Source: CAD feature listing. Evaluate the final solid. Frame: model axes, mm. Face numbers are marked on the shaded views. A direction names the side the tool comes from. Coordinates: 2 decimals unless noted, no trailing zeros. Order: outer loops, then holes, each group sorted by start corner. A loop starts at its lowest first (then second) coordinate and runs counter-clockwise, first axis right, second up. Notation, with made-up numbers: (31.5, 68.25) -> (57.5, 68.25) arc R16 ccw to (57.5, 78.25) -> close; hole circle Ø8 at (53.25, -34.75). An arc over 180 degrees is marked (long way). Put each result on its own line as item: value.
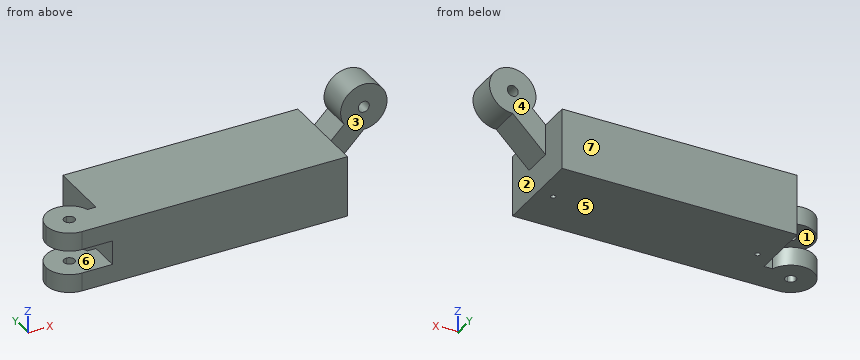
from build123d import *

# Parameters (mm, degrees)
SKETCH1_W           = 48.881284
SKETCH1_H           = 19.05
BOSS_EXTRUDE2_DEPTH = 12.7
BOSS_EXTRUDE3_DEPTH = 3.836458333
LPATTERN1_COUNT     = 2
LPATTERN1_PITCH     = 8.863541667
BOSS_EXTRUDE5_START = -9.525
SKETCH3_R           = 1.143
BOSS_EXTRUDE5_DEPTH = 3.175
SKETCH4_R           = 0.508
CUT_EXTRUDE1_DEPTH  = 7.62


with BuildPart() as part:
    # Sketch1 → Boss-Extrude2 (new body)
    with BuildSketch(Plane.XY):
        with Locations((24.440642, 9.525)):
            Rectangle(SKETCH1_W, SKETCH1_H)
    extrude(amount=BOSS_EXTRUDE2_DEPTH)

    # Sketch2 → Boss-Extrude3 (add)
    with BuildSketch(Plane(origin=(0, 0, 0), x_dir=(-1, 0, 0), z_dir=(0, 0, -1))):
        with BuildLine():
            ThreePointArc((1.77094988, 6.35), (2.435597108, 2.003283932), (6.35, 0))
            Line((6.35, 0), (6.35, 3.683))
            ThreePointArc((6.35, 3.683), (5.207, 4.826), (6.35, 5.969))
            Line((6.35, 5.969), (6.35, 6.35))
            Line((6.35, 6.35), (1.77094988, 6.35))
        make_face()
        with BuildLine():
            Line((6.35, 3.683), (6.35, 0))
            ThreePointArc((6.35, 0), (9.762497326, 1.413502674), (11.176, 4.826))
            ThreePointArc((11.176, 4.826), (7.121939156, 9.589862502), (1.77094988, 6.35))
            Line((1.77094988, 6.35), (6.35, 6.35))
            Line((6.35, 6.35), (6.35, 5.969))
            ThreePointArc((6.35, 5.969), (7.158223051, 5.634223051), (7.493, 4.826))
            ThreePointArc((7.493, 4.826), (7.158223051, 4.017776949), (6.35, 3.683))
        make_face()
        with BuildLine():
            Line((0, 6.35), (0, 0))
            Line((0, 0), (6.35, 0))
            ThreePointArc((6.35, 0), (2.435597108, 2.003283932), (1.77094988, 6.35))
            Line((1.77094988, 6.35), (0, 6.35))
        make_face()
    boss_extrude3 = extrude(amount=-BOSS_EXTRUDE3_DEPTH)

    # LPattern1: Boss-Extrude3 ×2
    with Locations(*[(0, 0, i * LPATTERN1_PITCH) for i in range(1, LPATTERN1_COUNT)]):
        add(boss_extrude3)

    # Sketch3 → Boss-Extrude5 (add, symmetric)
    with BuildSketch(Plane.XZ.offset(BOSS_EXTRUDE5_START)):
        with BuildLine():
            Line((51.617945235, 15.436661235), (48.881284, 12.7))
            Line((48.881284, 12.7), (48.881284, 6.35))
            Line((48.881284, 6.35), (55.706278652, 13.174994652))
            ThreePointArc((55.706278652, 13.174994652), (58.04238684, 22.223893483), (51.617945235, 15.436661235))
        make_face()
        with Locations(Location((55.706278652, 18.000994652, 0), (0, 0, 270))):
            Circle(SKETCH3_R, mode=Mode.SUBTRACT)
    extrude(amount=BOSS_EXTRUDE5_DEPTH, both=True)

    # Sketch4 → Cut-Extrude1 (cut)
    with BuildSketch(Plane(origin=(0, 0, 0), x_dir=(-1, 0, 0), z_dir=(0, 0, -1))):
        with Locations((-45.579284, 9.525)):
            Circle(SKETCH4_R)
        with Locations((-3.067304, 9.525)):
            Circle(SKETCH4_R)
    extrude(amount=-CUT_EXTRUDE1_DEPTH, mode=Mode.SUBTRACT)


solid = part.part
1. Cut plane A-A on y = 15. Output: boundary loops of the cut face in (x, z), plus the area to 3 significant figures.
Numbers:
outline: (0, 0) -> (48.88, 0) -> (48.88, 12.7) -> (0, 12.7) -> close
area: 621 mm2
2. Cut plane B-B on x = 23. Output: boundary loops of the cut face in (y, z), plus the area to 3 significant figures.
Numbers:
outline: (0, 0) -> (19.05, 0) -> (19.05, 12.7) -> (0, 12.7) -> close
area: 242 mm2
3. Set-up query: the marked faces 1, 2, 3 and 4. Return all of +Z, -Z, +X, -X, +Y, -Y with unobstructed straight access to the full face (end or side cutting, diameter ignored); none if empty.
Numbers:
face 1: -X, +Y, -Y
face 2: -Z, +X
face 3: +Z, -Z, +X, -Y
face 4: +Z, -Z, +X, +Y
4. First-contact query: pin 1 (5 mm diameter, centred on x = -6.5, y = 3.5, fed in from +Z); pin 2 (10 mm diameter, centred on y = 10.5, z = 4.5, fed in from +X); pin 3 (4 mm diameter, centred on x = 53.5, y = 4, fed in from -Z); pin 4 (6 mm diameter, centred on x = 56, z = 15, fed in from -Y). Flat tips, straight axial feed; report the tip coordinate or a pass-through.
Numbers:
pin 1: stops at z = 12.7
pin 2: stops at x = 52.03
pin 3: passes through
pin 4: stops at y = 6.35
5. Pull-direction query (Z, two-part tool) for the marked faces 5, 6 and 7; classes: pulls with the +Z half, pulls with the -Z half, needs draft (parallel to the pull), parting line crosses it, or undercut.
Numbers:
face 5: pulls with the -Z half
face 6: undercut
face 7: needs draft
6. Ray query, line 1 along Y through (x, z) = (3, 4.5); line 2 along Z through (x, y) = (10, 9.75); line 3 along X through (y, z) = (12.75, 10.5). Return the intervals inside material, ascending.
Numbers:
line 1: y = 0 to 9.02, 10.03 to 19.05
line 2: z = 0 to 12.7
line 3: x = 0 to 48.88
